Answer from the drawing. Dimensions are ordinates in mm from the lowest x, y and z of the part. Give positions to 0.01 mm unless a question says otherwise; leave off trailing zeros. Write each loop counter-clockwise with the first axis right and the second up, starting at its lowest first coordinate (ties: lowest second). Pieces come first, ordered by that corner, then holes. Notation, with made-up numbers: (-15.75, 40.25) - (-9.75, 40.25) arc R33 ccw to (-9.75, 70.25) - close; hole circle Ø3 at (10.25, 74). An arc over 180 degrees is marked (long way). Answer as a JSON object with one key per item and string values. Group by question number.
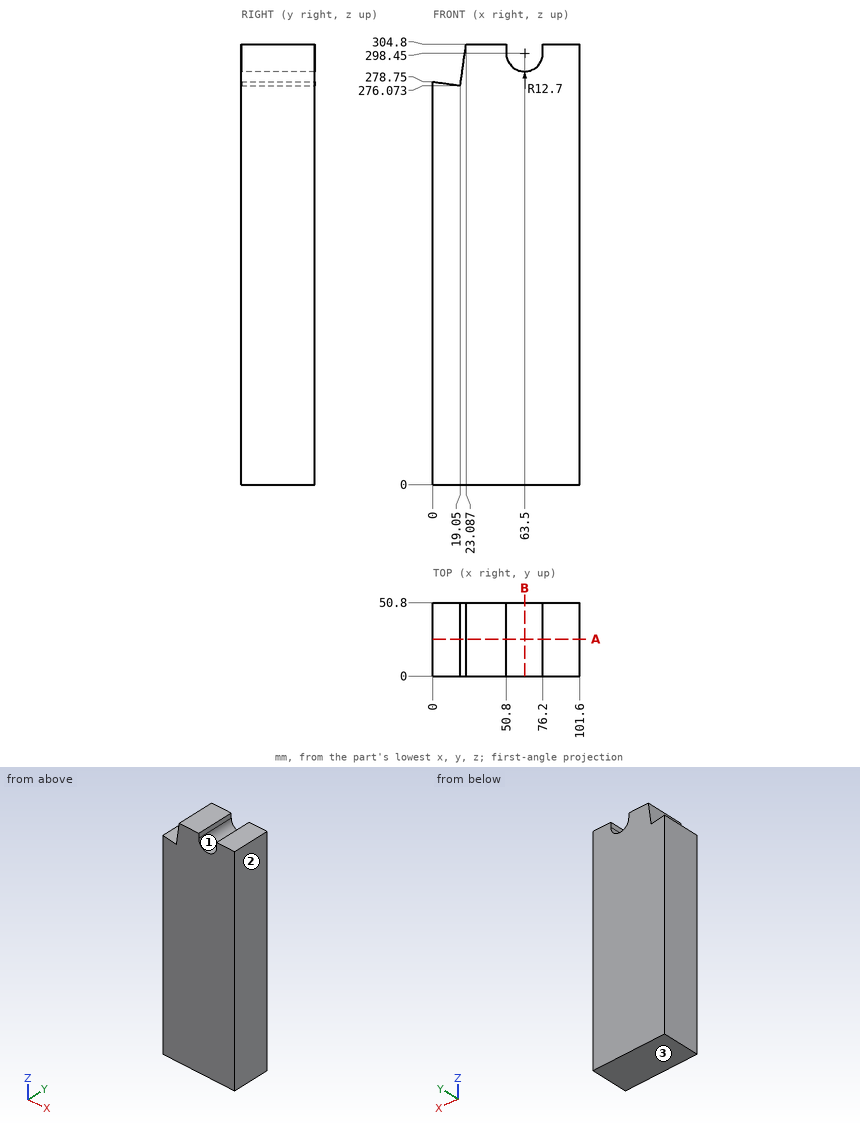
1) Flat-ended cylindrical pins translate along their axes: pin 1 Ø4 at (x, y) = (82.5, 39.5) entering from -Z; pin 2 Ø5 at (y, z) = (31, 301.5) entering from -X. Find the tip coordinate at first contact, or state that the pin passes through.
2) Find section B-B, the plane x = 63.5. Write down the section's boundary in (y, z).
3) Find section A-A, the plane y = 25.5. Write down the section's boundary in (x, z).
4) For a pull along X with two mould halves and no side action, classify the marked faces 1, 2 and 3 as released by +X, released by -X, zero draft, split by the parting line, or undercut.
5) Find the intervals of material crossed by line 1 (Z direction, x = 8.5, y = 44.5) (1 decimal); line 2 (Z direction, x = 54, y = 8.5), in increasing order. Write a range as [from, to].
Values follow:
{
 "1": {"pin 1": "stops at z = 0", "pin 2": "stops at x = 22.27"},
 "2": {"outline": "(0, 0) - (50.8, 0) - (50.8, 285.75) - (0, 285.75) - close"},
 "3": {"outline": "(0, 0) - (101.6, 0) - (101.6, 304.8) - (76.2, 304.8) - (76.2, 298.45) arc R12.7 cw to (50.8, 298.45) - (50.8, 304.8) - (23.09, 304.8) - (19.05, 276.07) - (0, 278.75) - close"},
 "4": {"face 1": "undercut", "face 2": "released by +X", "face 3": "zero draft"},
 "5": {"line 1": "z = [0, 277.6]", "line 2": "z = [0, 290.02]"}
}
